The listing builds one solid part. Answer for the finished solid, in the listing's coordinates (mm). Face numbers are marked on the shaded views. A direction names the side the tool comes from. Coordinates: 2 decimals unless noted, no trailing zeros. Loops run counter-clockwise (first coordinate to the right, second up) from the corner with the lowest first, then second, coordinate; pieces in that order, holes last. Notation, with made-up numbers: (4.25, -10.5) -> (61.25, -10.5) arc R31 cw to (61.25, 28.5) -> close; hole circle Ø3 at (-31.75, -12). An arc over 180 degrees is marked (long way). Answer in a Markdown table with one row per item.
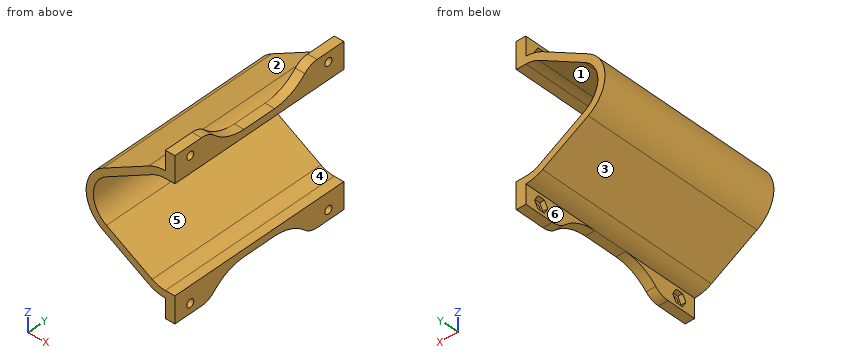
Autodesk Inventor part; units mm, degrees
ref_plane "YZ Plane" through (0, 0, 0) normal (1, 0, 0) x (0, 1, 0)
ref_plane "XZ Plane" through (0, 0, 0) normal (0, 1, 0) x (-1, 0, 0)
ref_plane "XY Plane" through (0, 0, 0) normal (0, 0, 1) x (1, 0, 0)
sketch "Эскиз1" plane through (0, 0, 0) normal (0, 1, 0) x (-1, 0, 0)
  circle A0 centre (0, 0) radius 11
  circle A1 centre (0, -22) radius 11
  circle A2 centre (19.0526, -11) radius 11
  line L0 (0, 0) -> (7, 12.1244)
  line L1 (0, 0) -> (14, 0) construction
  line L2 (0, -22) -> (7, -34.1244)
  line L3 (0, -22) -> (14, -22) construction
  line L4 (5.5, 9.5263) -> (24.5526, -1.4737)
  line L5 (5.5, -31.5263) -> (24.5526, -20.5263)
  circle A3 centre (0, 0) radius 14
  circle A4 centre (0, -22) radius 14
  circle A5 centre (19.0526, -11) radius 14
  line L6 (7, 12.1244) -> (26.0526, 1.1244)
  line L7 (7, -34.1244) -> (26.0526, -23.1244)
  line L8 (-14, 0) -> (-9, 0)
  line L9 (0, 11) -> (8.6603, 11) construction
  line L10 (0, 14) -> (-9, 14)
  line L11 (0, 11) -> (-9, 11)
  line L12 (0, -36) -> (-9, -36)
  line L13 (0, -33) -> (-9, -33)
  line L14 (-9, -36) -> (-9, 14)
  line L15 (-9, 11) -> (-6, 11)
  line L16 (-6, 11) -> (-6, 22)
  line L17 (-6, 22) -> (-9, 22)
  line L18 (-9, 22) -> (-9, 11)
  line L19 (-9, -33) -> (-6, -33)
  line L20 (-6, -33) -> (-6, -44)
  line L21 (-6, -44) -> (-9, -44)
  line L22 (-9, -44) -> (-9, -33)
  line L23 (-9, 11) -> (-4, 11)
  line L24 (-4, 11) -> (0, 11)
  line L25 (0, 11) -> (0, 22)
  line L26 (0, 22) -> (-4, 22)
  line L27 (-4, 22) -> (-4, 11)
  line L28 (-9, -33) -> (-4, -33)
  line L29 (-4, -33) -> (0, -33)
  line L30 (0, -33) -> (0, -44)
  line L31 (0, -44) -> (-4, -44)
  line L32 (-4, -44) -> (-4, -33)
  line L33 (-4, 11) -> (-4, -36)
  point P0 (-6, -36)
  point P1 (-6, 14)
  dimension "d10" = 22
  dimension "d12" = 22
  dimension "d13" = 14
  dimension "d14" = 60
  dimension "d15" = 14
  dimension "d16" = 60
  dimension "d17" = 28
  dimension "d20" = 9
  dimension "d21" = 3
  dimension "d22" = 11
  dimension "d23" = 3
  dimension "d24" = 11
  dimension "d53" = 5
  dimension "d54" = 4
  dimension "d55" = 5
extrude "Выдавливание1" add sketch "Эскиз1" along normal blind 77 contours A0 L25 A3 L0 | L0 A3 L4 | L11 L27 A3 L25 | L6 A5 L4 A3 | A3 L27 L10 | L10 L27 L26 L25 | A5 L5 A2 L4 | L7 A4 L5 A5 | A4 L30 A1 L2 | L2 L5 A4 | L12 L32 A4 | L30 L31 L32 L12 | A4 L32 L13 L30
sketch "Эскиз6" plane through (4, 0, -33) normal (1, 0, 0) x (0, 0, -1)
  line L0 (11, 0) -> (11, 77)
  line L1 (11, 0) -> (11, 31.5)
  line L2 (11, 77) -> (11, 45.5)
  line L3 (-47, 0) -> (-55, 0)
  line L4 (-55, 0) -> (-55, 31.5)
  line L5 (-55, 0) -> (-55, 77)
  line L6 (-55, 77) -> (-55, 45.5)
  line L7 (-47, 0) -> (-47, 77)
  line L8 (-55, 45.5) -> (-47, 45.5)
  line L9 (-47, 45.5) -> (-47, 31.5)
  line L10 (-47, 31.5) -> (-55, 31.5)
  line L11 (-55, 31.5) -> (-55, 45.5)
  line L12 (3, 0) -> (3, 77)
  line L13 (11, 31.5) -> (3, 31.5)
  line L14 (3, 31.5) -> (3, 45.5)
  line L15 (3, 45.5) -> (11, 45.5)
  line L16 (11, 45.5) -> (11, 31.5)
  arc A0 (3, 31.5) -> (11, 15.75) centre (22.9984, 31.7512) ccw
  arc A1 (11, 61.25) -> (3, 45.5) centre (22.9984, 45.2488) ccw
  arc A2 (-47, 45.5) -> (-55, 61.25) centre (-66.9984, 45.2488) ccw
  arc A3 (-55, 15.75) -> (-47, 31.5) centre (-66.9984, 31.7512) ccw
  point P0 (-33, 0)
  point P1 (3, 31.5)
  point P2 (11, 15.75)
  dimension "d56" = 31.5
  dimension "d57" = 31.5
  dimension "d58" = 31.5
  dimension "d59" = 31.5
  dimension "d60" = 20
  dimension "d61" = 20
  dimension "d62" = 20
  dimension "d63" = 20
extrude "Выдавливание5" cut sketch "Эскиз6" against normal blind 4 contours A0 L13 L0 | L13 L12 L15 L0 | L15 A1 L0 | L10 L5 L8 L7 | A3 L4 L10 | L8 L5 A2
fillet "Сопряжение2" radius 8 4 edges at (2, 15.75, -44) (2, 61.25, -44) (2, 61.25, 22) (2, 15.75, 22)
sketch "Эскиз7" plane through (0, 0, 14) normal (-1, 0, 0) x (0, 0, 1)
  line L0 (8, 0) -> (8, 12.1537)
  line L1 (8, 0) -> (4, 0)
  line L2 (8, 7) -> (8, 0)
  line L3 (4, 7) -> (-54, 7)
  line L4 (-54, 7) -> (-54, 70)
  line L5 (-54, 70) -> (4, 70)
  line L6 (4, 70) -> (4, 7)
  line L7 (4, 7) -> (1.4, 7)
  line L8 (-54, 70) -> (-51.4, 70)
  line L9 (1.4, 7) -> (-51.4, 7)
  line L10 (-51.4, 7) -> (-51.4, 70)
  line L11 (-51.4, 70) -> (1.4, 70)
  line L12 (1.4, 70) -> (1.4, 7)
  line L13 (1.4, 8.5011) -> (4, 10.0022)
  line L14 (4, 10.0022) -> (6.6, 8.5011)
  line L15 (6.6, 8.5011) -> (6.6, 5.4989)
  line L16 (6.6, 5.4989) -> (4, 3.9978)
  line L17 (4, 3.9978) -> (1.4, 5.4989)
  line L18 (1.4, 5.4989) -> (1.4, 8.5011)
  line L19 (-51.4, 5.4989) -> (-54, 3.9978)
  line L20 (-54, 3.9978) -> (-56.6, 5.4989)
  line L21 (-56.6, 5.4989) -> (-56.6, 8.5011)
  line L22 (-56.6, 8.5011) -> (-54, 10.0022)
  line L23 (-54, 10.0022) -> (-51.4, 8.5011)
  line L24 (-51.4, 8.5011) -> (-51.4, 5.4989)
  line L25 (-51.4, 68.4989) -> (-54, 66.9978)
  line L26 (-54, 66.9978) -> (-56.6, 68.4989)
  line L27 (-56.6, 68.4989) -> (-56.6, 71.5011)
  line L28 (-56.6, 71.5011) -> (-54, 73.0022)
  line L29 (-54, 73.0022) -> (-51.4, 71.5011)
  line L30 (-51.4, 71.5011) -> (-51.4, 68.4989)
  line L31 (1.4, 71.5011) -> (4, 73.0022)
  line L32 (4, 73.0022) -> (6.6, 71.5011)
  line L33 (6.6, 71.5011) -> (6.6, 68.4989)
  line L34 (6.6, 68.4989) -> (4, 66.9978)
  line L35 (4, 66.9978) -> (1.4, 68.4989)
  line L36 (1.4, 68.4989) -> (1.4, 71.5011)
  point P0 (-14, 0)
  point P1 (1.4, 68.4989)
  point P2 (1.4, 8.5011)
  dimension "d69" = 58
  dimension "d70" = 63
  dimension "d71" = 2.6
  dimension "d72" = 2.6
extrude "Выдавливание6" cut sketch "Эскиз7" against normal blind 2 contours L6 L14 L15 L16 L17 L18 L3 | L3 L12 L13 L6 | L24 L19 L20 L21 L22 L4 L3 | L3 L4 L23 L10 | L35 L12 L5 L6 | L6 L5 L36 L31 L32 L33 L34 | L25 L4 L5 L10 | L26 L27 L28 L29 L30 L5 L4
sketch "Эскиз8" plane through (2, 0, 14) normal (-1, 0, 0) x (0, 0, 1)
  line L0 (4, 7) -> (-54, 7)
  line L1 (-54, 7) -> (-54, 70)
  line L2 (-54, 70) -> (4, 70)
  line L3 (4, 70) -> (4, 7)
  circle A0 centre (4, 7) radius 1.6
  circle A1 centre (-54, 7) radius 1.6
  circle A2 centre (-54, 70) radius 1.6
  circle A3 centre (4, 70) radius 1.6
  point P0 (-14, 0)
  dimension "d75" = 3.2
  dimension "d76" = 3.2
  dimension "d77" = 3.2
  dimension "d78" = 3.2
extrude "Выдавливание7" cut sketch "Эскиз8" against normal blind 2 contours A1 L1 L0 | L0 L1 A1 | A0 L3 L0 | L0 L3 A0 | A2 L2 L1 | L1 L2 A2 | A3 L2 L3 | L3 L2 A3
sketch "Эскиз9" plane through (0, 77, 0) normal (0, 1, 0) x (1, 0, 0)
  point P0 (0, 0)
properties part number "battery_1"
Item 1: A cutting plane is placed at A-A, the plane x = -22. Determine the outline of the cut face in (y, z), plus the area to 3 significant figures.
Findings below:
| item | result |
|---|---|
| outline | (0, -25.46) -> (77, -25.46) -> (77, -22) -> (0, -22) -> close; (0, 0) -> (77, 0) -> (77, 3.46) -> (0, 3.46) -> close |
| area | 533 mm2 |
Item 2: A cutting plane is placed at B-B, the plane y = 7. Count the separate pieces of the cut face and the enclosed holes in it, plus the area to 3 significant figures.
Findings below:
| item | result |
|---|---|
| separate pieces | 3 |
| enclosed holes | 0 |
| area | 304 mm2 |
Item 3: A cutting plane is placed at D-D, the plane y = 23.5. Determine the outline of the cut face in (x, z), plus the area to 3 significant figures.
Findings below:
| item | result |
|---|---|
| outline | (-26.05, -23.12) -> (-7, -34.12) arc R14 ccw to (0, -36) -> (0, -37.78) -> (4, -37.78) -> (4, -33) -> (0, -33) arc R11 cw to (-5.5, -31.53) -> (-24.55, -20.53) arc R11 cw to (-24.55, -1.47) -> (-5.5, 9.53) arc R11 cw to (0, 11) -> (4, 11) -> (4, 15.78) -> (0, 15.78) -> (0, 14) arc R14 ccw to (-7, 12.12) -> (-26.05, 1.12) arc R14 ccw to start |
| area | 288 mm2 |
Item 4: Find the intervals of material crossed by probe 1 along Z at (x, y) = (3.45, 70); probe 2 along Y at (x, z) = (2.4, -40); probe 3 along Z at (x, y) = (-18, 17.5), in increasing order.
Findings below:
| item | result |
|---|---|
| probe 1 | z = -44 to -41.6, -38.4 to -33, 11 to 16.4, 19.6 to 22 |
| probe 2 | y = 0 to 5.4, 8.6 to 19.75, 57.25 to 68.4, 71.6 to 77 |
| probe 3 | z = -27.77 to -24.31, 2.31 to 5.77 |
Item 5: A cutting plane is placed at C-C, the plane z = 2.5. Determine the outline of the cut face in (x, y).
Findings below:
| item | result |
|---|---|
| outline | (-23.67, 0) -> (-17.67, 0) -> (-17.67, 77) -> (-23.67, 77) -> close |
Item 6: Flat-ended cylindrical pins translate along their axes: pin 1 Ø2.5 at (y, z) = (70, -41.5) entering from -X; pin 2 Ø3.5 at (y, z) = (7, -40) entering from -X; pin 3 Ø10 at (x, z) = (-13.5, 7.5) entering from -Y; pin 4 Ø1.5 at (x, y) = (-25, 29) entering from -Z. Find the tip coordinate at first contact, or state that the pin passes through.
Findings below:
| item | result |
|---|---|
| pin 1 | stops at x = 0 |
| pin 2 | stops at x = 2 |
| pin 3 | stops at y = 0 |
| pin 4 | stops at z = -24.17 |
Item 7: A tool of negligible diameter and unlimited length cuts with its end or side. For the marked faces 1 and 2, from which of +Z, -Z, +X, -X, +Y, -Y can it reach the whole face along a straight path? Write none if from no direction.
Findings below:
| item | result |
|---|---|
| face 1 | +X, +Y, -Y |
| face 2 | +Z, -X, +Y, -Y |
Item 8: Determine the mould class of the marked faces 3, 4, 5 and 6 for opening direction Z: +Z half, -Z half, draft (parallel to the pull), parting line (faces both ways), or undercut.
Findings below:
| item | result |
|---|---|
| face 3 | -Z half |
| face 4 | undercut |
| face 5 | undercut |
| face 6 | draft |
